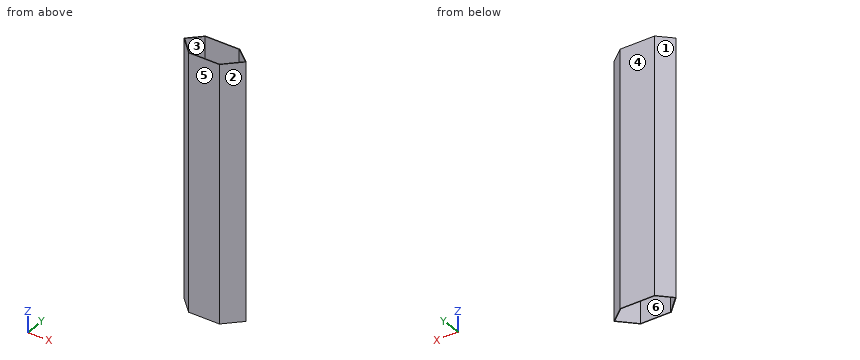
from build123d import *

# Parameters (mm, degrees)
F1_DEPTH = 210


with BuildPart() as f1:
    # F0 (on Top) → F1 (new body)
    with BuildSketch(Plane.XY):
        Polygon((-54.881843, 7.859512), (-42.890312, -2.118638), (-55.363, -14.591326), (-55.861931, -15.091326), (-55.155894, -15.091326), (-42.149323, -2.084756), (-54.701024, 8.359512), (-83.010021, 8.359512), (-93.488171, -2.118638), (-80.515483, -15.091326), (-79.807307, -15.091326), (-80.308376, -14.591326), (-92.781064, -2.118638), (-82.802914, 7.859512), align=None)
        Polygon((-55.861931, -15.091326), (-55.363, -14.591326), (-80.308376, -14.591326), (-79.807307, -15.091326), align=None)
    extrude(amount=F1_DEPTH)


solid = f1.part
For this review, take the finished solid that the model builds, in its own axes (mm). Face numbers are marked on the shaded views. A direction names the side the tool comes from. Round coordinates to 2 decimals unless told otherwise and drop trailing zeros. Write each loop counter-clockwise with the first axis right and the second up, starting at its lowest first coordinate (ties: lowest second). Pieces come first, ordered by that corner, then holes. Notation, with made-up numbers: (-16, 81) -> (39, 81) arc R23 cw to (39, 112) -> close; hole circle Ø10 at (58, -13). An arc over 180 degrees is marked (long way). Use CSV: the item, a comma, the result in double quotes.
(1) Consider section A-A, the plane z = 50. Give the boundary of the cut face in (x, y).
Computed values:
outline,"(-93.49, -2.12) -> (-80.52, -15.09) -> (-55.16, -15.09) -> (-42.15, -2.08) -> (-54.7, 8.36) -> (-83.01, 8.36) -> close; hole (-92.78, -2.12) -> (-80.31, -14.59) -> (-55.36, -14.59) -> (-42.89, -2.12) -> (-54.88, 7.86) -> (-82.8, 7.86) -> close"
(2) Consider section B-B, the plane x = -76. Give the boundary of the cut face in (y, z), plus the area to 3 significant figures.
Computed values:
outline,"(-15.09, 0) -> (-14.59, 0) -> (-14.59, 210) -> (-15.09, 210) -> close; (7.86, 0) -> (8.36, 0) -> (8.36, 210) -> (7.86, 210) -> close"
area,"210 mm²"
(3) To check wall thickness, follow L1, parallel to Y at x = -67, z = 90; L2, parallel to X at y = -7.5, z = 13.5; L3, parallel to X at y = 1.5, z = 122. State the ranges of each line that lie inside material, in increasing order. Write a range as [from, to].
Computed values:
L1,"[-15.09, -14.59], [7.86, 8.36]"
L2,"[-88.11, -87.4], [-48.27, -47.56]"
L3,"[-89.87, -89.16], [-47.24, -46.46]"
(4) For the marked faces 5 and 6, list the 3-axis set-ups (+Z, -Z, +X, -X, +Y, -Y) from which the entire face can be reached by the end or side of a thin tool; tool diameter is ignored.
Computed values:
face 5,"+Z, -Z, +X, -X, -Y"
face 6,"+Z, -Z"
(5) Consider section C-C, the plane y = 1. Give the boundary of the cut face in (x, z).
Computed values:
outline,"(-90.37, 0) -> (-89.66, 0) -> (-89.66, 210) -> (-90.37, 210) -> close; (-46.64, 0) -> (-45.86, 0) -> (-45.86, 210) -> (-46.64, 210) -> close"
(6) Clearance check with flat-ended pins moving along their axes: P1, Ø8, axis at y = -3, z = 31, coming from the +X side; P2, Ø2, axis at y = 2, z = 133.5, coming from the +X side; P3, Ø8, axis at y = -8.5, z = 182, coming from the +X side. State where each tip first meets the part, or that it passes through.
Computed values:
P1,"x = -42.15"
P2,"x = -45.86"
P3,"x = -44.56"
(7) Draft analysis for pull direction X (two halves, no side actions). For the marked faces 1, 2, 3 and 4, state which applies: +X half, -X half, draft (parallel to the pull), parting line (faces both ways), or undercut.
Computed values:
face 1,"-X half"
face 2,"+X half"
face 3,"undercut"
face 4,"draft"
